Autodesk Fusion 360 part; units mm, degrees
sketch "Sketch1" plane through (0, 0, 0) normal (0, 1, 0) x (1, 0, 0)
  circle A0 centre (0, 0) radius 33.075
  circle A1 centre (0, 0) radius 35
  dimension "d1" = 66.15
  dimension "d2" = 70
extrude "Extrude1" add sketch "Sketch1" along normal blind 7 contours A0
extrude "Extrude2" add sketch "Sketch1" against normal blind 2 contours A0 | A1
sketch "Sketch4" plane through (0, -2, 0) normal (0, -1, 0) x (1, 0, 0)
  circle A0 centre (0, 0) radius 35
  circle A1 centre (14, 0) radius 10.5
  circle A2 centre (0, 0) radius 33.075
  dimension "d33" = 21
  dimension "d39" = 14
extrude "Extrude8" cut sketch "Sketch4" against normal up to surface (9 mm away) contours A1
sketch "Sketch5" plane through (0, 7, 0) normal (0, 1, 0) x (-1, 0, 0)
  circle A0 centre (-14, 0) radius 10.5
  circle A1 centre (0, 0) radius 33.075
  circle A2 centre (-14, 0) radius 13.25
  dimension "d36" = 26.5
extrude "Extrude9" cut sketch "Sketch5" against normal blind 7 contours A2
mirror "Mirror3" about plane through (0, 0, 0) normal (1, 0, 0) of "Extrude9", "Extrude8"
Design review of the part built by this model. Coordinates are the model's own, in mm. A direction names the side the tool comes from. Coordinates: 2 decimals unless noted, no trailing zeros. Order: outer loops, then holes, each group sorted by start corner. A loop starts at its lowest first (then second) coordinate and runs counter-clockwise, first axis right, second up.
Item 1: Take a section at D-D, the plane z = 22.5. Write out the cut boundary in (x, y).
Item 2: Take a section at A-A, the plane z = 0. Write out the cut boundary in (x, y) (3 decimals).
Item 3: Take a section at C-C, the plane y = 4.5. Write out the cut boundary in (x, z) (3 decimals).
Item 4: For pin 1 Ø4 at (y, z) = (3.5, 12.5) entering from +X; pin 2 Ø2 at (x, y) = (-8, -0.5) entering from -Z; pin 3 Ø3 at (y, z) = (4, -23) entering from -X, all flat-tipped, find the tip position at first contact; note any pin that passes through.
Item 5: For line 1 (X direction, y = 6.25, z = -1); line 2 (X direction, y = 0.25, z = -6.5); line 3 (Z direction, x = 8, y = 3.5), list the stretches that pass through material, from the lowest coordinate up.
Item 6: The part is to be moulded in two halves that separate along Z. For faces 3 (the cylindrical face through (31.55, 3.45, 9.93)), 4 (the flat face through (26, 0, -21)), 5 (the cylindrical face through (-1.36, 3.55, -3.98)), say which applies: pulls with the +Z half, pulls with the -Z half, needs draft (parallel to the pull), parting line crosses it, or undercut.
Item 7: For faces 1 (the flat face through (18, 0, 10)), 2 (the cylindrical face through (-28, -1, 21)), list the 3-axis set-ups (+Z, -Z, +X, -X, +Y, -Y) from which the entire face can be reached by the end or side of a thin tool; tool diameter is ignored.
Item 8: Take a section at B-B, the plane x = 9.5. Write out the cut boundary in (y, z).
The answers:
1. outline: (-26.81, -2) - (26.81, -2) - (26.81, 0) - (24.24, 0) - (24.24, 7) - (-24.24, 7) - (-24.24, 0) - (-26.81, 0) - close
2. outline: (-35, -2) - (-24.5, -2) - (-24.5, 0) - (-27.25, 0) - (-27.25, 7) - (-33.075, 7) - (-33.075, 0) - (-35, 0) - close; (-3.5, -2) - (3.5, -2) - (3.5, 0) - (0.75, 0) - (0.75, 7) - (-0.75, 7) - (-0.75, 0) - (-3.5, 0) - close; (24.5, -2) - (35, -2) - (35, 0) - (33.075, 0) - (33.075, 7) - (27.25, 7) - (27.25, 0) - (24.5, 0) - close
3. outline: circle Ø66.15 at (0, 0); hole circle Ø26.5 at (-14, 0); hole circle Ø26.5 at (14, 0)
4. pin 1: stops at x = 31.36
4. pin 2: stops at z = -34.29
4. pin 3: stops at x = -25.13
5. line 1: x = -33.06 to -27.21, -0.79 to 0.79, 27.21 to 33.06
5. line 2: x = -32.43 to -25.55, -2.45 to 2.45, 25.55 to 32.43
5. line 3: z = -32.09 to -11.81, 11.81 to 32.09
6. face 3: parting line crosses it
6. face 4: needs draft
6. face 5: undercut
7. face 1: +Y
7. face 2: +Y, -Y
8. outline: (-2, -33.69) - (0, -33.69) - (0, -31.68) - (7, -31.68) - (7, -12.46) - (0, -12.46) - (0, -9.49) - (-2, -9.49) - close; (-2, 9.49) - (0, 9.49) - (0, 12.46) - (7, 12.46) - (7, 31.68) - (0, 31.68) - (0, 33.69) - (-2, 33.69) - close
